The drawing under review shows one solid part. Ordinate dimensions are in mm from its lowest x, y, z. A direction names the side the tool comes from. Give positions to 0.01 mm unless a question says otherwise; leave off trailing zeros. Order: outer loops, then holes, each group sorted by start corner. A loop starts at its lowest first (then second) coordinate and runs counter-clockwise, first axis right, second up. Notation, with made-up numbers: (-14, 30) -> (-8, 30) arc R19 ccw to (-8, 55) -> close; hole circle Ø4 at (75.25, -29.75). An arc over 180 degrees is marked (long way). One line per item, written item: value.
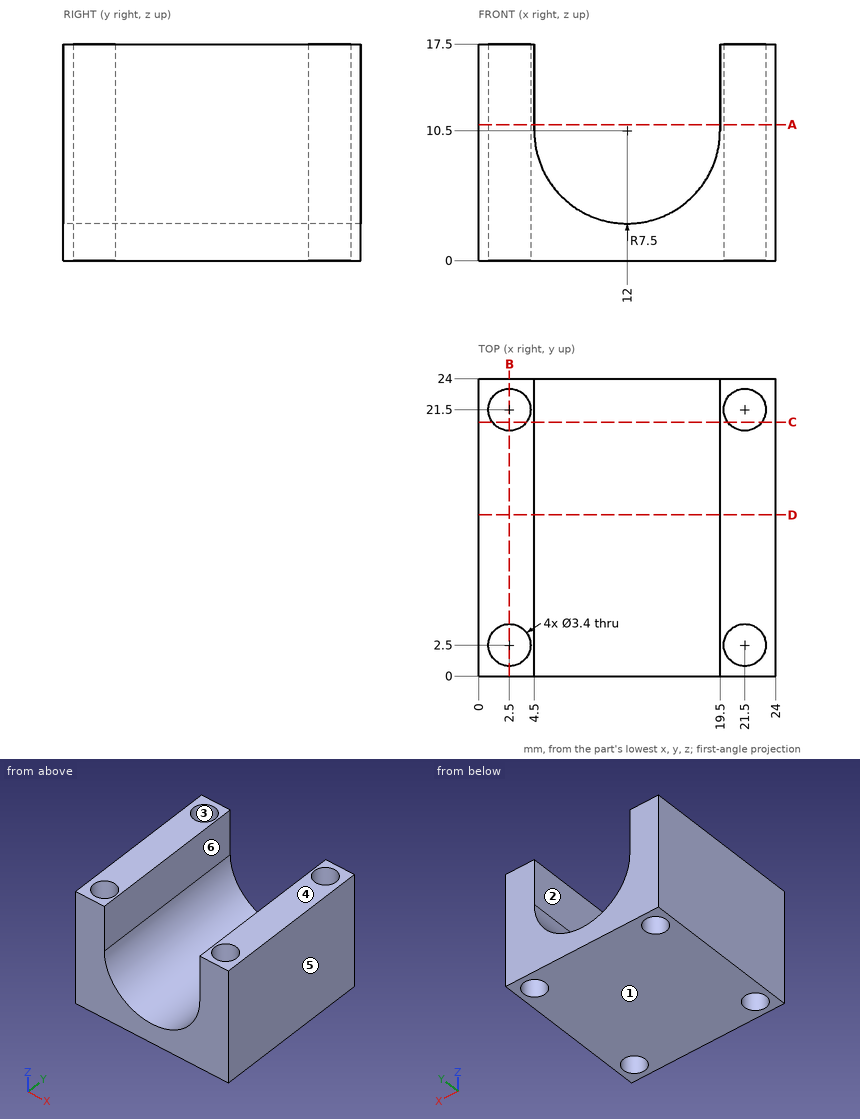
Item 1: Draft analysis for pull direction X (two halves, no side actions). For the marked faces 3, 4, 5 and 6, state which applies: pulls with the +X half, pulls with the -X half, needs draft (parallel to the pull), parting line crosses it, or undercut.
Returned:
face 3: undercut
face 4: needs draft
face 5: pulls with the +X half
face 6: undercut
Item 2: Add section D-D on y = 13. Give the boundary of the cut face in (x, z), plus the area to 3 significant figures.
Returned:
outline: (0, 0) -> (24, 0) -> (24, 17.5) -> (19.5, 17.5) -> (19.5, 10.5) arc R7.5 cw to (4.5, 10.5) -> (4.5, 17.5) -> (0, 17.5) -> close
area: 227 mm²
Item 3: Add section B-B on x = 2.5. Give the boundary of the cut face in (y, z).
Returned:
outline: (0, 0) -> (0.8, 0) -> (0.8, 17.5) -> (0, 17.5) -> close; (4.2, 0) -> (19.8, 0) -> (19.8, 17.5) -> (4.2, 17.5) -> close; (23.2, 0) -> (24, 0) -> (24, 17.5) -> (23.2, 17.5) -> close
Item 4: To check wall thickness, follow line 1 along Y through (x, z) = (21.5, 3.5); line 2 along X through (y, z) = (10, 14.25); line 3 along X through (y, z) = (21.5, 9.25). State the ranges of each line that lie inside material, in increasing order. Write a range as from..to.
Returned:
line 1: 0..0.8, 4.2..19.8, 23.2..24
line 2: 0..4.5, 19.5..24
line 3: 0..0.8, 4.2..4.6, 19.4..19.8, 23.2..24
Item 5: Clearance check with flat-ended pins moving along their axes: P1, Ø3, axis at x = 21.5, y = 21.5, coming from the +Z side; P2, Ø5, axis at x = 12.5, y = 18.5, coming from the +Z side; P3, Ø10, axis at x = 12.5, y = 14.5, coming from the +Z side. State where each tip first meets the part, or that it passes through.
Returned:
P1: through
P2: z = 3.63
P3: z = 5.4
Item 6: Machinability: for the marked faces 1 and 2, which of the approach directions +Z, -Z, +X, -X, +Y, -Y give a long, thin tool a straight path to every point of the face, cutting with its end or side? Answer none if there is none.
Returned:
face 1: -Z, +X, -X, +Y, -Y
face 2: +Z, +Y, -Y
Item 7: Add section C-C on y = 20.5. Give the boundary of the cut face in (x, z), plus the area to 3 significant figures.
Returned:
outline: (0, 0) -> (1.13, 0) -> (1.13, 17.5) -> (0, 17.5) -> close; (3.87, 0) -> (20.13, 0) -> (20.13, 17.5) -> (19.5, 17.5) -> (19.5, 10.5) arc R7.5 cw to (4.5, 10.5) -> (4.5, 17.5) -> (3.87, 17.5) -> close; (22.87, 0) -> (24, 0) -> (24, 17.5) -> (22.87, 17.5) -> close
area: 130 mm²
Item 8: Add section A-A on z = 11. Give the boundary of the cut face in (x, y), plus the area to 3 significant figures.
Returned:
outline: (0, 0) -> (4.5, 0) -> (4.5, 24) -> (0, 24) -> close; (19.5, 0) -> (24, 0) -> (24, 24) -> (19.5, 24) -> close; hole circle Ø3.4 at (2.5, 2.5); hole circle Ø3.4 at (2.5, 21.5); hole circle Ø3.4 at (21.5, 2.5); hole circle Ø3.4 at (21.5, 21.5)
area: 180 mm²
